```python
from build123d import *

# Parameters (mm, degrees)
SKETCH_1_W          = 42
SKETCH_1_H          = 42
EXTRUDE_1_DEPTH     = 5
SKETCH_2_W          = 42
SKETCH_2_H          = 5
EXTRUDE_2_DEPTH     = 3
SKETCH_4_W          = 5
SKETCH_4_H          = 42
EXTRUDE_3_DEPTH     = 25
SKETCH_5_W          = 3
SKETCH_5_H          = 42
EXTRUDE_4_DEPTH     = 42
SKETCH_8_R          = 7.5
CUT_EXTRUDE_1_DEPTH = 25


with BuildPart() as part:
    # 草图1 → 凸台-拉伸1 (new body)
    with BuildSketch(Plane(origin=(0, 0, 0), x_dir=(1, 0, 0), z_dir=(0, 1, 0))):
        Rectangle(SKETCH_1_W, SKETCH_1_H)
    extrude(amount=EXTRUDE_1_DEPTH)

    # 草图2 → 凸台-拉伸2 (add)
    with BuildSketch(Plane.ZY.offset(21)):
        with Locations((0, 2.5)):
            Rectangle(SKETCH_2_W, SKETCH_2_H)
    extrude(amount=EXTRUDE_2_DEPTH)

    # 草图4 → 凸台-拉伸3 (add)
    with BuildSketch(Plane(origin=(0, 5, 0), x_dir=(1, 0, 0), z_dir=(0, 1, 0))):
        with Locations((-21.5, 0)):
            Rectangle(SKETCH_4_W, SKETCH_4_H)
    extrude(amount=EXTRUDE_3_DEPTH)

    # 草图5 → 凸台-拉伸4 (add)
    with BuildSketch(Plane.XZ):
        with Locations((-22.5, 0)):
            Rectangle(SKETCH_5_W, SKETCH_5_H)
    extrude(amount=EXTRUDE_4_DEPTH)

    # 草图8 → 切除-拉伸1 (cut)
    with BuildSketch(Plane(origin=(0, 5, 0), x_dir=(1, 0, 0), z_dir=(0, 1, 0))):
        with Locations(Location((0, 0, 0), (0, 0, 270))):
            Circle(SKETCH_8_R)
    extrude(amount=-CUT_EXTRUDE_1_DEPTH, mode=Mode.SUBTRACT)


solid = part.part
```
Source: CAD feature listing. Evaluate the final solid. Frame: model axes, mm. A direction names the side the tool comes from. Round coordinates to 2 decimals unless told otherwise and drop trailing zeros. Loops run counter-clockwise (first coordinate to the right, second up) from the corner with the lowest first, then second, coordinate; pieces in that order, holes last. Notation, with made-up numbers: M 14,89 L 56,89 A13 cw 56,112 Z; hole C 44,50 d9. An arc over 180 degrees is marked long. Use a Markdown table: item, result. Add a question column.
1. Set-up query: faces 4 (the flat face through (-13, 2, -21)), 5 (the flat face through (-19, 17, 0)), 6 (the flat face through (-21, -21, 0)). Return all of +Z, -Z, +X, -X, +Y, -Y with unobstructed straight access to the full face (end or side cutting, diameter ignored); none if empty.
2. Cut plane C-C, the plane z = 14. Output: boundary loops of the cut face in (x, y).
3. Cut plane B-B, the plane x = 0. Output: boundary loops of the cut face in (y, z).
4. Cut plane D-D, the plane y = -30. Output: boundary loops of the cut face in (x, z).
5. Cut plane A-A, the plane z = 0. Output: boundary loops of the cut face in (x, y), and give its area (3 significant figures).
6. Contact query for flat-ended pins moving along their axis: pin 1 (10 mm diameter, centred on x = -12, z = -7.5, fed in from +Y); pin 2 (7.5 mm diameter, centred on y = 14, z = 0, fed in from +X); pin 3 (21 mm diameter, centred on x = -3.5, z = 8, fed in from -Y); pin 4 (5 mm diameter, centred on x = -2, z = 1.5, fed in from -Y). Output: stop coordinate, or through.
7. Pull-direction query (Z, two-part tool) for faces 1 (the cylindrical face through (0.33, 2.535, -7.493)), 2 (the flat face through (-24, -5, 0)), 3 (the flat face through (-13, 2, 21)); classes: +Z half, -Z half, draft (parallel to the pull), parting line (faces both ways), or undercut.
8. Ray query, line 1 along X through (y, z) = (3, 0); line 2 along Z through (x, y) = (-0.5, 4); line 3 along X through (y, z) = (-32, 13.5). Return the intervals inside material, ascending. Write a range as [from, to].
Solution:
| question | item | result |
|---|---|---|
| 1 | face 4 | -Z, +X, -X, +Y, -Y |
| 1 | face 5 | +Z, -Z, +X, +Y |
| 1 | face 6 | +Z, -Z, +X, -Y |
| 2 | outline | M -24,-42 L -21,-42 L -21,0 L 21,0 L 21,5 L -19,5 L -19,30 L -24,30 Z |
| 3 | outline | M 0,-21 L 5,-21 L 5,-7.5 L 0,-7.5 Z; M 0,7.5 L 5,7.5 L 5,21 L 0,21 Z |
| 4 | outline | M -24,-21 L -21,-21 L -21,21 L -24,21 Z |
| 5 | outline | M -24,-42 L -21,-42 L -21,0 L -7.5,0 L -7.5,5 L -19,5 L -19,30 L -24,30 Z; M 7.5,0 L 21,0 L 21,5 L 7.5,5 Z |
| 5 | area | 401 mm2 |
| 6 | pin 1 | stops at y = 5 |
| 6 | pin 2 | stops at x = -19 |
| 6 | pin 3 | stops at y = 0 |
| 6 | pin 4 | passes through |
| 7 | face 1 | undercut |
| 7 | face 2 | draft |
| 7 | face 3 | +Z half |
| 8 | line 1 | x = [-24, -7.5], [7.5, 21] |
| 8 | line 2 | z = [-21, -7.48], [7.48, 21] |
| 8 | line 3 | x = [-24, -21] |
